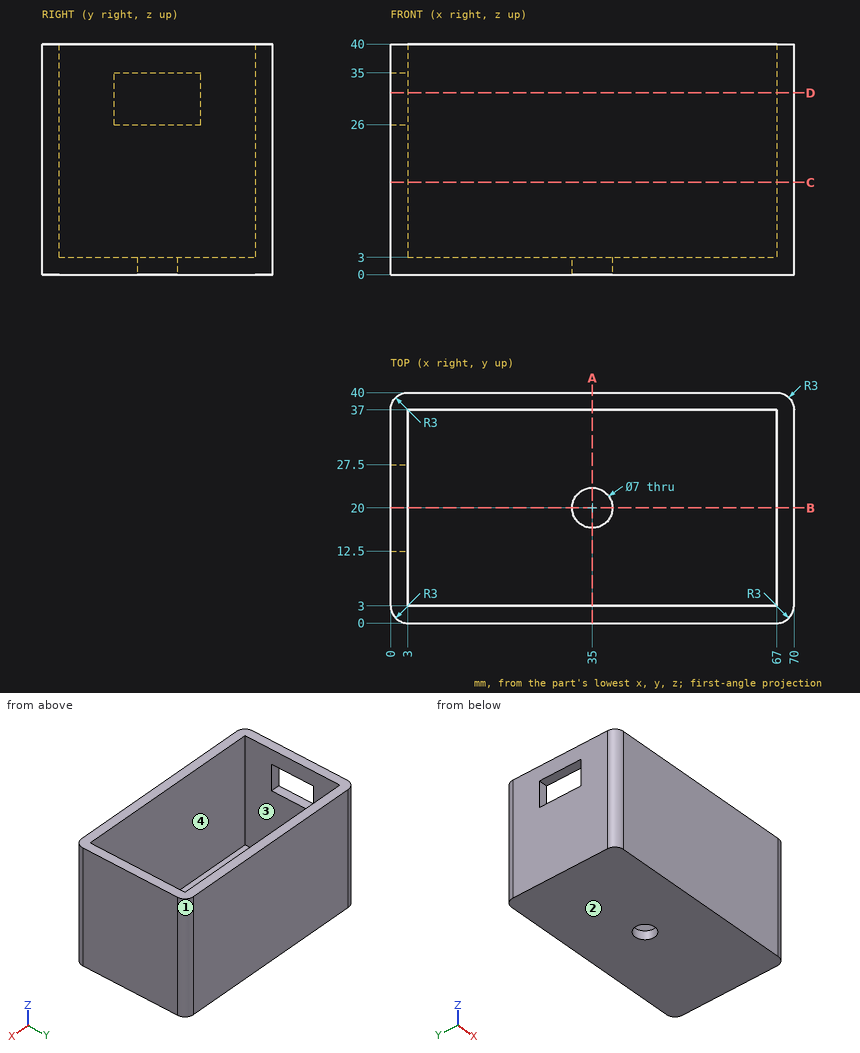
Geometry: see drawing. Coordinates: mm, zero at the bounding-box minimum. Coordinates: 2 decimals unless noted, no trailing zeros. Order: outer loops, then holes, each group sorted by start corner. A loop starts at its lowest first (then second) coordinate and runs counter-clockwise, first axis right, second up. Notation, with made-up numbers: (-35, 47) - (7, 47) arc R3 cw to (7, 51) - close; hole circle Ø6 at (11.25, -36). An arc over 180 degrees is marked (long way). Write each question's results on one line, items separated by ' | '.
(1) First-contact query: pin 1 Ø1.5 at (x, z) = (2, 31.5) entering from -Y; pin 2 Ø2 at (x, y) = (50, 30) entering from +Z. Flat tips, straight axial feed; report the tip coordinate or a pass-through.
Values found:
pin 1: stops at y = 0.01 | pin 2: stops at z = 3
(2) Mould query, pull axis X, two halves, no side actions, for the marked faces 1, 2, 3 and 4. Classes: +X half, -X half, draft (parallel to the pull), parting line (faces both ways), or undercut.
Values found:
face 1: +X half | face 2: draft | face 3: undercut | face 4: undercut
(3) Section query C-C, the plane z = 16. Return the cut outline in (x, y).
Values found:
outline: (0, 3) arc R3 ccw to (3, 0) - (67, 0) arc R3 ccw to (70, 3) - (70, 37) arc R3 ccw to (67, 40) - (3, 40) arc R3 ccw to (0, 37) - close; hole (3, 3) - (67, 3) - (67, 37) - (3, 37) - close
(4) Section query D-D, the plane z = 31.5. Return the cut outline in (x, y), plus the area to 3 significant figures.
Values found:
outline: (0, 3) arc R3 ccw to (3, 0) - (67, 0) arc R3 ccw to (70, 3) - (70, 37) arc R3 ccw to (67, 40) - (3, 40) arc R3 ccw to (0, 37) - (0, 27.5) - (3, 27.5) - (3, 37) - (67, 37) - (67, 3) - (3, 3) - (3, 12.5) - (0, 12.5) - close | area: 571 mm²
(5) Section query A-A, the plane x = 35. Return the cut outline in (y, z).
Values found:
outline: (0, 0) - (16.5, 0) - (16.5, 3) - (3, 3) - (3, 40) - (0, 40) - close; (23.5, 0) - (40, 0) - (40, 40) - (37, 40) - (37, 3) - (23.5, 3) - close
(6) Section query B-B, the plane y = 20. Return the cut outline in (x, z).
Values found:
outline: (0, 0) - (31.5, 0) - (31.5, 3) - (3, 3) - (3, 26) - (0, 26) - close; (0, 35) - (3, 35) - (3, 40) - (0, 40) - close; (38.5, 0) - (70, 0) - (70, 40) - (67, 40) - (67, 3) - (38.5, 3) - close
(7) Line query: line 1 (Y direction, x = 35, z = 2.2); line 2 (Y direction, x = 62.5, z = 16); line 3 (X direction, y = 31, z = 38). Output: solid intervals per line, ascending. Write a range as [from, to].
Values found:
line 1: y = [0, 16.5], [23.5, 40] | line 2: y = [0, 3], [37, 40] | line 3: x = [0, 3], [67, 70]
